```python
from build123d import *

# Parameters (mm, degrees)
SKETCH017_W     = 171.4
SKETCH017_H     = 216.7
PAD008_DEPTH    = 7
SKETCH020_W     = 61.167203
SKETCH020_H     = 139
POCKET010_DEPTH = 2
POCKET011_DEPTH = 6
SKETCH022_W     = 24
SKETCH022_H     = 138.401909
POCKET012_DEPTH = 5
POCKET014_DEPTH = 1.9
POCKET015_DEPTH = 7
POCKET016_DEPTH = 6.5
POCKET017_DEPTH = 5.5
SKETCH029_W     = 6.217281
SKETCH029_H     = 19.8
POCKET018_DEPTH = 4.5
SKETCH031_W     = 23.945183
SKETCH031_H     = 46.145969
POCKET020_DEPTH = 25
SKETCH033_W     = 12.346496
SKETCH033_H     = 29.812275
POCKET022_DEPTH = 4
SKETCH036_R     = 1.95
POCKET025_DEPTH = 5
SKETCH039_R     = 1.95
POCKET028_DEPTH = 5
SKETCH_W        = 27.295079
SKETCH_H        = 2
SKETCH_W_2      = 27.490026
SKETCH_W_3      = 28.268842
SKETCH_W_4      = 27.05204
PAD_DEPTH       = 1
SKETCH049_R     = 9.5
POCKET030_DEPTH = 3.5
SKETCH053_R     = 4.25
POCKET033_DEPTH = 2.4
SKETCH054_R     = 1.95
POCKET034_DEPTH = 15
SKETCH055_W     = 15.4
SKETCH055_H     = 4.4
SKETCH055_W_2   = 4.4
SKETCH055_H_2   = 15.4
POCKET035_DEPTH = 4.4
SKETCH057_W     = 4
SKETCH057_H     = 6
POCKET036_DEPTH = 2
SKETCH060_R     = 1.95
POCKET038_DEPTH = 5


with BuildPart() as part:
    # Sketch017 → Pad008 (new body)
    with BuildSketch(Plane(origin=(0, 0, -8), x_dir=(-1, 0, 0), z_dir=(0, 0, -1))):
        with Locations((-6.555, 0)):
            Rectangle(SKETCH017_W, SKETCH017_H)
    extrude(amount=-PAD008_DEPTH)

    # Sketch020 (on DatumPlane) → Pocket010 (cut)
    with BuildSketch(Plane.XY.offset(-1)):
        with Locations((78.757783, 0)):
            Rectangle(SKETCH020_W, SKETCH020_H)
    extrude(amount=-POCKET010_DEPTH, mode=Mode.SUBTRACT)

    # Sketch021 (on DatumPlane) → Pocket011 (cut)
    with BuildSketch(Plane.XY.offset(-1)):
        with BuildLine():
            ThreePointArc((60, 78.009018), (58.828427, 80.837445), (56, 82.009018))
            Line((37.5, 82.009018), (56, 82.009018))
            ThreePointArc((37.5, 82.009018), (34.671573, 80.837445), (33.5, 78.009018))
            Line((33.5, 40.652546), (33.5, 78.009018))
            ThreePointArc((33.5, 40.652546), (34.671573, 37.824119), (37.5, 36.652546))
            Line((56, 36.652546), (37.5, 36.652546))
            ThreePointArc((56, 36.652546), (58.828427, 37.824119), (60, 40.652546))
            Line((60, 78.009018), (60, 40.652546))
        make_face()
    extrude(amount=-POCKET011_DEPTH, mode=Mode.SUBTRACT)

    # Sketch022 (on DatumPlane) → Pocket012 (cut)
    with BuildSketch(Plane(origin=(0, 0, -8), x_dir=(1, 0, 0), z_dir=(0, 0, -1))):
        with Locations((15.400889, -30.961346)):
            Rectangle(SKETCH022_W, SKETCH022_H)
    extrude(amount=-POCKET012_DEPTH, mode=Mode.SUBTRACT)

    # Sketch025 (on DatumPlane) → Pocket014 (cut)
    with BuildSketch(Plane.XY.offset(-1)):
        with BuildLine():
            Line((93.246833, -69.304718), (61.387916, -69.304718))
            Line((61.387916, -69.304718), (55.011108, -64.243446))
            Line((55.011108, -64.243446), (41.330532, -64.243446))
            Line((41.330532, -64.243446), (41.330532, -102.943491))
            ThreePointArc((41.330532, -102.943491), (44.021527, -106.897224), (48.686769, -105.844145))
            Line((48.686769, -105.844145), (53.077853, -101.141844))
            Line((53.077853, -101.141844), (93.246833, -101.141844))
            Line((93.246833, -101.141844), (93.246833, -69.304718))
        make_face()
    extrude(amount=-POCKET014_DEPTH, mode=Mode.SUBTRACT)

    # Sketch026 (on DatumPlane) → Pocket015 (cut)
    with BuildSketch(Plane.XY.offset(-1)):
        Polygon((41.572746, -79.724867), (88.10059, -79.724867), (88.10059, -99.524867), (50.134747, -99.524867), (49.401962, -100.487076), (41.572746, -100.487076), (41.572746, -99.426659), align=None)
    extrude(amount=-POCKET015_DEPTH, mode=Mode.SUBTRACT)

    # Sketch027 (on DatumPlane) → Pocket016 (cut)
    with BuildSketch(Plane.XY.offset(-1)):
        with BuildLine():
            ThreePointArc((-4.121528, -40.918728), (-6.949955, -42.090301), (-8.121528, -44.918728))
            Line((-8.121528, -102.988314), (-8.121528, -44.918728))
            ThreePointArc((-8.121528, -102.988314), (-6.949955, -105.816741), (-4.121528, -106.988314))
            Line((45.499925, -106.988314), (-4.121528, -106.988314))
            ThreePointArc((45.499925, -106.988314), (48.328352, -105.816741), (49.499925, -102.988314))
            Line((49.499925, -44.918728), (49.499925, -102.988314))
            ThreePointArc((49.499925, -44.918728), (48.328352, -42.090301), (45.499925, -40.918728))
            Line((-4.121528, -40.918728), (45.499925, -40.918728))
        make_face()
    extrude(amount=-POCKET016_DEPTH, mode=Mode.SUBTRACT)

    # Sketch028 (on DatumPlane) → Pocket017 (cut)
    with BuildSketch(Plane.XY.offset(-1)):
        Polygon((3.400889, -29.656117), (27.400889, -29.656117), (27.400889, -41.656117), (3.400889, -41.797379), align=None)
    extrude(amount=-POCKET017_DEPTH, mode=Mode.SUBTRACT)

    # Sketch029 (on DatumPlane) → Pocket018 (cut)
    with BuildSketch(Plane.XY.offset(-1)):
        with Locations((91.20923, -89.624867)):
            Rectangle(SKETCH029_W, SKETCH029_H)
    extrude(amount=-POCKET018_DEPTH, mode=Mode.SUBTRACT)

    # Sketch031 (on DatumPlane) → Pocket020 (cut)
    with BuildSketch(Plane.XY.offset(-1)):
        with Locations((15.154121, -71.770674)):
            Rectangle(SKETCH031_W, SKETCH031_H)
        with BuildLine():
            Line((33.974045, -40.918728), (45.499925, -40.918728))
            ThreePointArc((49.499925, -44.918728), (48.328352, -42.090301), (45.499925, -40.918728))
            Line((49.499925, -44.918728), (49.499925, -69.331493))
            Line((49.499925, -69.331493), (33.974045, -69.331493))
            Line((33.974045, -69.331493), (33.974045, -40.918728))
        make_face()
    extrude(amount=-POCKET020_DEPTH, mode=Mode.SUBTRACT)

    # Sketch033 (on DatumPlane) → Pocket022 (cut)
    with BuildSketch(Plane(origin=(0, 0, -8), x_dir=(1, 0, 0), z_dir=(0, 0, -1))):
        with Locations((29.792881, -58.674055)):
            Rectangle(SKETCH033_W, SKETCH033_H)
    extrude(amount=-POCKET022_DEPTH, mode=Mode.SUBTRACT)

    # Sketch036 (on Face3 of Pad008) → Pocket025 (cut)
    with BuildSketch(Plane.XZ.offset(108.35)):
        with Locations((-68.2, -4.5)):
            Circle(SKETCH036_R)
        with Locations((84.8, -4.5)):
            Circle(SKETCH036_R)
    extrude(amount=-POCKET025_DEPTH, mode=Mode.SUBTRACT)

    # Sketch039 (on Face1 of Pad008) → Pocket028 (cut)
    with BuildSketch(Plane(origin=(0, 108.35, 0), x_dir=(-1, 0, 0), z_dir=(0, 1, 0))):
        with Locations((-84.8, -4.5)):
            Circle(SKETCH039_R)
        with Locations((68.2, -4.5)):
            Circle(SKETCH039_R)
    extrude(amount=-POCKET028_DEPTH, mode=Mode.SUBTRACT)

    # Sketch (on DatumPlane) → Pad (join)
    with BuildSketch(Plane(origin=(0, 0, -8), x_dir=(1, 0, 0), z_dir=(0, 0, -1))):
        with Locations((16.35246, 23)):
            Rectangle(SKETCH_W, SKETCH_H)
        with Locations((16.254987, -9)):
            Rectangle(SKETCH_W_2, SKETCH_H)
        with Locations((15.865579, -41)):
            Rectangle(SKETCH_W_3, SKETCH_H)
        with Locations((16.47398, -79)):
            Rectangle(SKETCH_W_4, SKETCH_H)
    extrude(amount=-PAD_DEPTH)

    # Sketch049 (on DatumPlane) → Pocket030 (cut)
    with BuildSketch(Plane(origin=(0, 0, -8), x_dir=(1, 0, 0), z_dir=(0, 0, -1))):
        with Locations((-67, -90)):
            Circle(SKETCH049_R)
        with Locations((80, -90)):
            Circle(SKETCH049_R)
        with Locations((80, 70)):
            Circle(SKETCH049_R)
        with Locations((-67, 70)):
            Circle(SKETCH049_R)
    extrude(amount=-POCKET030_DEPTH, mode=Mode.SUBTRACT)

    # Sketch053 (on DatumPlane) → Pocket033 (cut)
    with BuildSketch(Plane(origin=(0, 0, -8), x_dir=(1, 0, 0), z_dir=(0, 0, -1))):
        with Locations((-70, 0)):
            Circle(SKETCH053_R)
        with Locations((-4, 0)):
            Circle(SKETCH053_R)
        with Locations((70, 104.200928)):
            Circle(SKETCH053_R)
        with Locations((-70, 96.649681)):
            Circle(SKETCH053_R)
        with Locations((67.474617, -100)):
            Circle(SKETCH053_R)
        with Locations((-54.612518, -100)):
            Circle(SKETCH053_R)
    extrude(amount=-POCKET033_DEPTH, mode=Mode.SUBTRACT)

    # Sketch054 (on DatumPlane) → Pocket034 (cut)
    with BuildSketch(Plane(origin=(0, 0, -8), x_dir=(1, 0, 0), z_dir=(0, 0, -1))):
        with Locations((-70, 96.649681)):
            Circle(SKETCH054_R)
        with Locations((70, 104.170845)):
            Circle(SKETCH054_R)
        with Locations((-4, 0)):
            Circle(SKETCH054_R)
        with Locations((-70, 0)):
            Circle(SKETCH054_R)
        with Locations((-54.612518, -100)):
            Circle(SKETCH054_R)
        with Locations((67.474617, -100)):
            Circle(SKETCH054_R)
    extrude(amount=-POCKET034_DEPTH, mode=Mode.SUBTRACT)

    # Sketch055 (on DatumPlane) → Pocket035 (cut)
    with BuildSketch(Plane(origin=(0, 0, -8), x_dir=(1, 0, 0), z_dir=(0, 0, -1))):
        with Locations((-39.835839, -92.167499)):
            Rectangle(SKETCH055_W, SKETCH055_H)
        with Locations((-52.2, 37.941446)):
            Rectangle(SKETCH055_W_2, SKETCH055_H_2)
        with Locations((-52.2, 12.541446)):
            Rectangle(SKETCH055_W_2, SKETCH055_H_2)
        with Locations((-52.2, -12.858554)):
            Rectangle(SKETCH055_W_2, SKETCH055_H_2)
        with Locations((-52.2, -38.258554)):
            Rectangle(SKETCH055_W_2, SKETCH055_H_2)
        with Locations((-14.435839, -92.167499)):
            Rectangle(SKETCH055_W, SKETCH055_H)
        with Locations((-50.851364, 98.832999)):
            Rectangle(SKETCH055_W, SKETCH055_H)
        with Locations((-25.451364, 98.832999)):
            Rectangle(SKETCH055_W, SKETCH055_H)
        with Locations((42.388664, 25.651083)):
            Rectangle(SKETCH055_W_2, SKETCH055_H_2)
        with Locations((42.388664, 0.251083)):
            Rectangle(SKETCH055_W_2, SKETCH055_H_2)
        with Locations((42.388664, -25.148917)):
            Rectangle(SKETCH055_W_2, SKETCH055_H_2)
        with Locations((78.951774, -74.70213)):
            Rectangle(SKETCH055_W, SKETCH055_H)
        with Locations((50.78279, -99.61552)):
            Rectangle(SKETCH055_W, SKETCH055_H)
    extrude(amount=-POCKET035_DEPTH, mode=Mode.SUBTRACT)

    # Sketch057 (on DatumPlane) → Pocket036 (cut)
    with BuildSketch(Plane(origin=(0, 0, -8), x_dir=(1, 0, 0), z_dir=(0, 0, -1))):
        with Locations((90.650505, 12)):
            Rectangle(SKETCH057_W, SKETCH057_H)
        with Locations((90.650505, -12)):
            Rectangle(SKETCH057_W, SKETCH057_H)
    extrude(amount=-POCKET036_DEPTH, mode=Mode.SUBTRACT)

    # Sketch060 (on DatumPlane) → Pocket038 (cut)
    with BuildSketch(Plane(origin=(-79.145, 0, 0), x_dir=(0, -1, 0), z_dir=(-1, 0, 0))):
        with Locations((-54.5, -4.5)):
            Circle(SKETCH060_R)
        with Locations((54.5, -4.5)):
            Circle(SKETCH060_R)
    extrude(amount=-POCKET038_DEPTH, mode=Mode.SUBTRACT)


solid = part.part
```
Build history of the part. All positions in model axes, mm. A direction names the side the tool comes from. Round coordinates to 2 decimals unless told otherwise and drop trailing zeros. Write each loop counter-clockwise with the first axis right and the second up, starting at its lowest first coordinate (ties: lowest second). Pieces come first, ordered by that corner, then holes. Notation, with made-up numbers: (20, -11.75) -> (37, -11.75) arc R10 ccw to (37, 7.25) -> close; hole circle Ø10 at (60.5, 48). An arc over 180 degrees is marked (long way). Put each result on its own line as item: value.
Item 1: Tool access for faces 1 (the face through (42, -17.951, -6)), 2 (the face through (70, 1, -3)): list every direction of +Z, -Z, +X, -X, +Y, -Y with a clear straight run to the whole face (end or side of a thin tool).
Here are the results:
face 1: -Z
face 2: +Z, +X
Item 2: Wall check: probe 1 along Y at (x, z) = (30, -5.25); probe 2 along X at (y, z) = (-28, -4.25) (3 decimals); probe 3 along X at (y, z) = (0, -6.9) (3 decimals). Give the ranges that are in metal, low to high. Write a range as from..to.
Here are the results:
probe 1: y = -108.35..-106.99, -40.92..43.77, 73.58..108.35
probe 2: x = -79.145..3.401, 27.401..40.189, 44.589..92.255
probe 3: x = -79.145..-74.25, -65.75..-8.25, 0.25..3.401, 27.401..40.189, 44.589..92.255
Item 3: Flat gauge pins, fed straight in: P1, Ø4, axis at y = 68.5, z = -2, coming from the +X side (3 decimals); P2, Ø7.5, axis at x = 70, y = -104.2, coming from the -Z side; P3, Ø1.2, axis at y = 54, z = -5, coming from the -X side (3 decimals). Where does each tip first touch, or does it go through?
Here are the results:
P1: stops at x = 92.255
P2: stops at z = -5.6
P3: stops at x = -74.145
Item 4: Slice it at A-A, the plane x = 80. Give the cut face in (y, z).
Here are the results:
outline: (-108.35, -8) -> (-99.52, -8) -> (-99.52, -2.9) -> (-101.14, -2.9) -> (-101.14, -1) -> (-108.35, -1) -> close; (-79.72, -8) -> (-79.5, -8) -> (-79.5, -4.5) -> (-60.5, -4.5) -> (-60.5, -8) -> (72.5, -8) -> (72.5, -3.6) -> (76.9, -3.6) -> (76.9, -8) -> (80.5, -8) -> (80.5, -4.5) -> (99.5, -4.5) -> (99.5, -8) -> (108.35, -8) -> (108.35, -1) -> (69.5, -1) -> (69.5, -3) -> (-69.5, -3) -> (-69.5, -2.9) -> (-79.72, -2.9) -> close
Item 5: Slice it at B-B, the plane y = -75. Give the cut face in (x, z) (3 decimals), plus the area to 3 significant figures.
Here are the results:
outline: (-79.145, -8) -> (-75.078, -8) -> (-75.078, -4.5) -> (-58.922, -4.5) -> (-58.922, -8) -> (3.182, -8) -> (3.182, -7.5) -> (-8.122, -7.5) -> (-8.122, -1) -> (-79.145, -1) -> close; (27.127, -8) -> (71.922, -8) -> (71.922, -4.5) -> (88.078, -4.5) -> (88.078, -8) -> (92.255, -8) -> (92.255, -2.9) -> (49.5, -2.9) -> (49.5, -7.5) -> (27.127, -7.5) -> close
area: 619 mm^2
Item 6: Two-plate mould, pull along Y, no slides. Class faces 3 (the face through (-65.946, -1.277, -6.817)), 4 (the face through (92.255, 23, -5)): pulls with the +Y half, pulls with the -Y half, needs draft (parallel to the pull), parting line crosses it, or undercut.
Here are the results:
face 3: undercut
face 4: needs draft
